Here's the drawing with two shaded views (mm, measured from the low corner). I have some questions. A direction names the side the tool comes from. Round coordinates to 2 decimals unless told otherwise and drop trailing zeros. Order: outer loops, then holes, each group sorted by start corner. A loop starts at its lowest first (then second) coordinate and runs counter-clockwise, first axis right, second up.
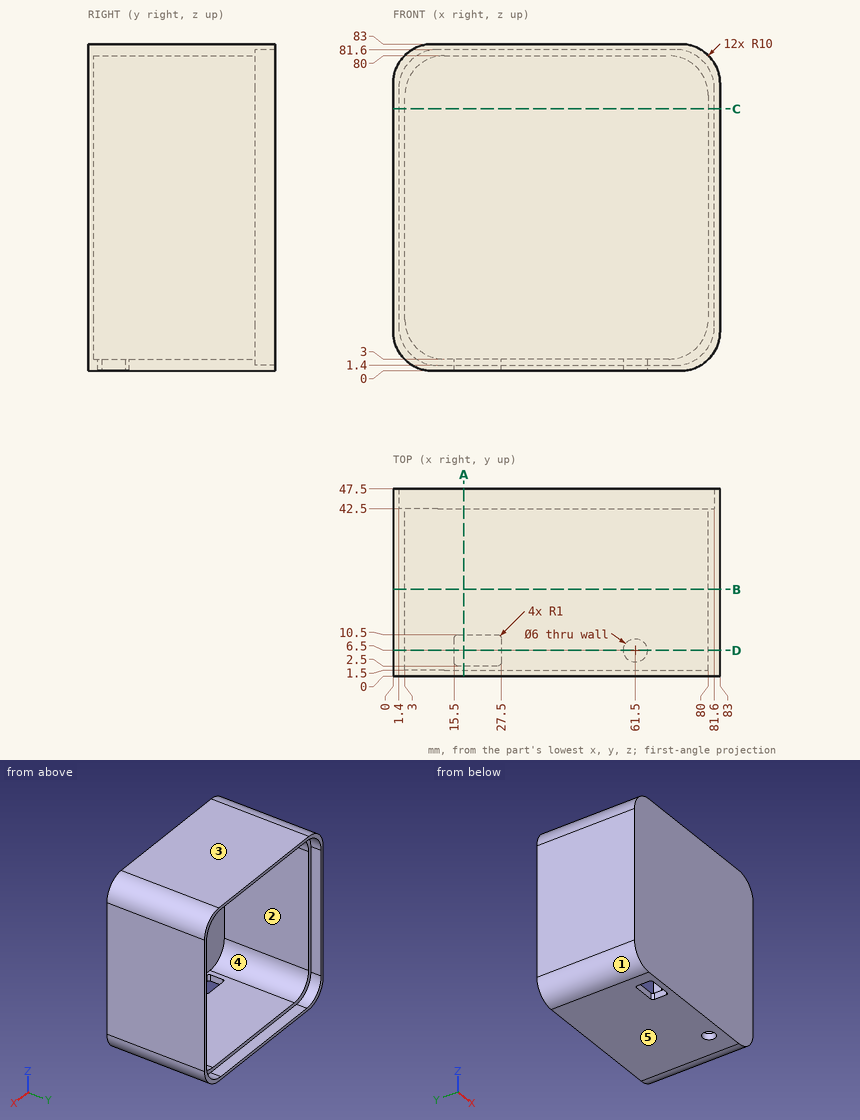
1. If we mould it in two halves opening along Z, with no side actions, what happens to the marked faces 1, 2 and 3? For each: released by +Z, released by -Z, zero draft, split by the parting line, or undercut.
Evaluation:
face 1: released by -Z
face 2: undercut
face 3: released by +Z
2. I need wall thicknesses on probe 1 along Z at (x, y) = (23.5, 44); probe 2 along Y at (x, z) = (61.5, 1.95); probe 3 along Y at (x, z) = (61.5, 1.25). Which ranges of each line are inside material? Lowest first, please.
Evaluation:
probe 1: z = 0 to 1.4, 81.6 to 83
probe 2: y = 0 to 3.5, 9.5 to 42.5
probe 3: y = 0 to 3.5, 9.5 to 47.5
3. I'm going to push flat-ended pins straight in: P1, Ø3.5, axis at y = 7.5, z = 1, coming from the +X side; P2, Ø1.5, axis at y = 7.5, z = 2, coming from the -X side; P3, Ø0.9, axis at x = 22, z = 2, coming from the +Y side. Where does each tip first touch, or does it pass through?
Evaluation:
P1: stops at x = 79.89
P2: stops at x = 3.11
P3: stops at y = 42.5
4. If we section it at A-A, the plane x = 18: Write out the boundary of the cut face in (y, z).
Evaluation:
outline: (0, 0) - (2.5, 0) - (2.5, 3) - (1.5, 3) - (1.5, 80) - (42.5, 80) - (42.5, 81.6) - (47.5, 81.6) - (47.5, 83) - (0, 83) - close; (10.5, 0) - (47.5, 0) - (47.5, 1.4) - (42.5, 1.4) - (42.5, 3) - (10.5, 3) - close
5. If we section it at C-C, the plane z = 66.5: Write out the boundary of the cut face in (x, y).
Evaluation:
outline: (0, 0) - (83, 0) - (83, 47.5) - (81.6, 47.5) - (81.6, 42.5) - (80, 42.5) - (80, 1.5) - (3, 1.5) - (3, 42.5) - (1.4, 42.5) - (1.4, 47.5) - (0, 47.5) - close
6. If we section it at B-B, the plane y = 22: Write out the boundary of the cut face in (x, z), and give its area (3 significant figures).
Evaluation:
outline: (0, 10) arc R10 ccw to (10, 0) - (73, 0) arc R10 ccw to (83, 10) - (83, 73) arc R10 ccw to (73, 83) - (10, 83) arc R10 ccw to (0, 73) - close; hole (3, 13) arc R10 ccw to (13, 3) - (70, 3) arc R10 ccw to (80, 13) - (80, 70) arc R10 ccw to (70, 80) - (13, 80) arc R10 ccw to (3, 70) - close
area: 960 mm2
7. On a 3-axis mill with a long thin cutter (end or side, diameter ignored), from which of +Z, -Z, +X, -X, +Y, -Y can I reach the whole of each face in a straight line? I mean the marked faces 4 and 5. Say none if no direction works.
Evaluation:
face 4: +Y
face 5: -Z, +X, -X, +Y, -Y
8. If we section it at D-D, the plane y = 6.5: Write out the boundary of the cut face in (x, z), and give its area (3 significant figures).
Evaluation:
outline: (0, 10) arc R10 ccw to (10, 0) - (15.5, 0) - (15.5, 3) - (13, 3) arc R10 cw to (3, 13) - (3, 70) arc R10 cw to (13, 80) - (70, 80) arc R10 cw to (80, 70) - (80, 13) arc R10 cw to (70, 3) - (64.5, 3) - (64.5, 0) - (73, 0) arc R10 ccw to (83, 10) - (83, 73) arc R10 ccw to (73, 83) - (10, 83) arc R10 ccw to (0, 73) - close; (27.5, 0) - (58.5, 0) - (58.5, 3) - (27.5, 3) - close
area: 906 mm2
